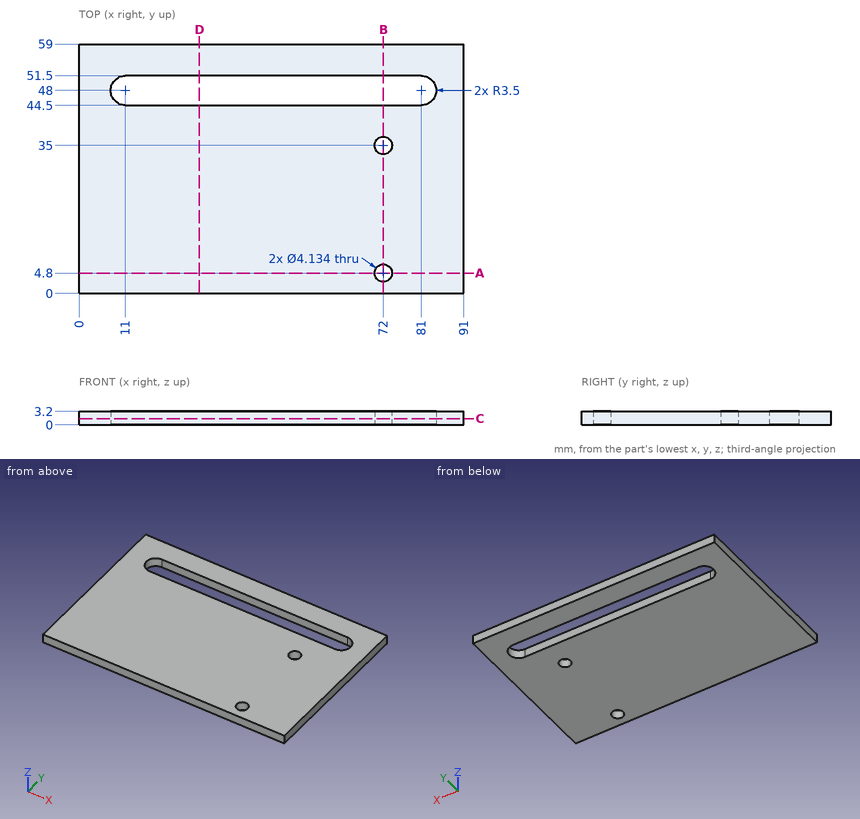
Geometry: see drawing. Coordinates: mm, zero at the bounding-box minimum. Give positions to 0.01 mm unless a question says otherwise; leave off trailing zeros. Write each loop counter-clockwise with the first axis right and the second up, starting at its lowest first coordinate (ties: lowest second). Pieces come first, ordered by that corner, then holes. Notation, with made-up numbers: (22, 51.25) - (68, 51.25) arc R8 cw to (68, 59.25) - close; hole circle Ø4 at (34.5, 10). An arc over 180 degrees is marked (long way). Return JSON: item names as keys, results as strings. Group by question number.
1) First-contact query: P1, Ø12, axis at x = 67.5, y = 37, coming from the -Z side. Flat tip, straight axial feed; report the tip coordinate or a pass-through.
2) Section A-A on y = 4.8. Return the cut outline in (x, z).
3) Section C-C on z = 1.5. Return the cut outline in (x, y).
4) Section D-D on x = 28.5. Return the cut outline in (y, z), plus the area to 3 significant figures.
5) Line query: line 1 (Y direction, x = 72, z = 2.3); line 2 (Y direction, x = 44, z = 2.2); line 3 (X direction, y = 35, z = 2.55). Output: solid intervals per line, ascending.
6) Section B-B on x = 72. Return the cut outline in (y, z).
Filled in:
{
 "1": {"P1": "stops at z = 0"},
 "2": {"outline": "(0, 0) - (69.93, 0) - (69.93, 3.2) - (0, 3.2) - close; (74.07, 0) - (91, 0) - (91, 3.2) - (74.07, 3.2) - close"},
 "3": {"outline": "(0, 0) - (91, 0) - (91, 59) - (0, 59) - close; hole (11, 44.5) - (81, 44.5) arc R3.5 ccw to (81, 51.5) - (11, 51.5) arc R3.5 ccw to start; hole circle Ø4.13 at (72, 4.8); hole circle Ø4.13 at (72, 35)"},
 "4": {"outline": "(0, 0) - (44.5, 0) - (44.5, 3.2) - (0, 3.2) - close; (51.5, 0) - (59, 0) - (59, 3.2) - (51.5, 3.2) - close", "area": "166 mm^2"},
 "5": {"line 1": "y = 0 to 2.73, 6.87 to 32.93, 37.07 to 44.5, 51.5 to 59", "line 2": "y = 0 to 44.5, 51.5 to 59", "line 3": "x = 0 to 69.93, 74.07 to 91"},
 "6": {"outline": "(0, 0) - (2.73, 0) - (2.73, 3.2) - (0, 3.2) - close; (6.87, 0) - (32.93, 0) - (32.93, 3.2) - (6.87, 3.2) - close; (37.07, 0) - (44.5, 0) - (44.5, 3.2) - (37.07, 3.2) - close; (51.5, 0) - (59, 0) - (59, 3.2) - (51.5, 3.2) - close"}
}
